```python
from build123d import *

# Parameters (mm, degrees)
SKETCH1_R           = 29
BOSS_EXTRUDE1_DEPTH = 3
SKETCH3_R           = 4
BOSS_EXTRUDE2_DEPTH = 4
SKETCH2_R           = 1.9
CUT_EXTRUDE1_DEPTH  = 42.605288125
SKETCH6_R           = 1.4
CUT_EXTRUDE3_DEPTH  = 10
SKETCH7_R           = 1.4
CUT_EXTRUDE4_DEPTH  = 10
CUT_EXTRUDE5_START  = -10
CUT_EXTRUDE5_DEPTH  = 10
SKETCH4_R           = 1.4
CUT_EXTRUDE7_DEPTH  = 10


with BuildPart() as part:
    # Sketch1 → Boss-Extrude1 (new body)
    with BuildSketch(Plane(origin=(0, 0, 0), x_dir=(1, 0, 0), z_dir=(0, 1, 0))):
        with Locations(Location((0, 0, 0), (0, 0, 270))):
            Circle(SKETCH1_R)
    extrude(amount=BOSS_EXTRUDE1_DEPTH)

    # Sketch3 → Boss-Extrude2 (add)
    with BuildSketch(Plane.XZ):
        with Locations(Location((0, 0, 0), (0, 0, 90))):
            Circle(SKETCH3_R)
    extrude(amount=BOSS_EXTRUDE2_DEPTH)

    # Sketch2 → Cut-Extrude1 (cut, through all)
    with BuildSketch(Plane(origin=(0, 3, 0), x_dir=(1, 0, 0), z_dir=(0, 1, 0))):
        with Locations(Location((0, 0, 0), (0, 0, 270))):
            Circle(SKETCH2_R)
    extrude(amount=-CUT_EXTRUDE1_DEPTH, mode=Mode.SUBTRACT)

    # Sketch6 → Cut-Extrude3 (cut)
    with BuildSketch(Plane(origin=(0, 3, 0), x_dir=(1, 0, 0), z_dir=(0, 1, 0))):
        with Locations(Location((26, 0, 0), (0, 0, 270))):
            Circle(SKETCH6_R)
        with Locations(Location((-26, 0, 0), (0, 0, 270))):
            Circle(SKETCH6_R)
    extrude(amount=-CUT_EXTRUDE3_DEPTH, mode=Mode.SUBTRACT)

    # Sketch7 → Cut-Extrude4 (cut)
    with BuildSketch(Plane(origin=(0, 3, 0), x_dir=(1, 0, 0), z_dir=(0, 1, 0))):
        with Locations(Location((-10, 21.451657064, 0), (0, 0, 270))):
            Circle(SKETCH7_R)
        with Locations(Location((10, 21.451657064, 0), (0, 0, 270))):
            Circle(SKETCH7_R)
    extrude(amount=-CUT_EXTRUDE4_DEPTH, mode=Mode.SUBTRACT)

    # Sketch7_3 → Cut-Extrude5 (cut)
    with BuildSketch(Plane(origin=(0, 3, 0), x_dir=(1, 0, 0), z_dir=(0, 1, 0)).offset(CUT_EXTRUDE5_START)):
        with BuildLine():
            Line((-14, 25.396850198), (0, 25.396850198))
            Line((0, 25.396850198), (0, 29))
            ThreePointArc((0, 29), (-7.228116776, 28.08477039), (-14, 25.396850198))
        make_face()
        with BuildLine():
            Line((0, 29), (0, 25.396850198))
            Line((0, 25.396850198), (14, 25.396850198))
            ThreePointArc((14, 25.396850198), (7.228116776, 28.08477039), (0, 29))
        make_face()
    extrude(amount=CUT_EXTRUDE5_DEPTH, mode=Mode.SUBTRACT)

    # Sketch4 → Cut-Extrude7 (cut)
    with BuildSketch(Plane(origin=(0, 3, 0), x_dir=(1, 0, 0), z_dir=(0, 1, 0))):
        with Locations(Location((-5, -22.025954195, 0), (0, 0, 270))):
            Circle(SKETCH4_R)
        with Locations(Location((5, -22.025954195, 0), (0, 0, 270))):
            Circle(SKETCH4_R)
    extrude(amount=-CUT_EXTRUDE7_DEPTH, mode=Mode.SUBTRACT)


solid = part.part
```
Source: CAD feature listing. Evaluate the final solid. Frame: model axes, mm. A direction names the side the tool comes from. Give positions to 0.01 mm unless a question says otherwise; leave off trailing zeros. Order: outer loops, then holes, each group sorted by start corner. A loop starts at its lowest first (then second) coordinate and runs counter-clockwise, first axis right, second up.
(1) Section query D-D (y = -3). Return the cut outline in (x, z).
(2) Section query A-A (z = 0). Return the cut outline in (x, y), plus the area to 3 significant figures.
(3) Contact query for flat-ended pins moving along their axis: P1, Ø3.5, axis at x = 5, z = 22.03, coming from the -Y side; P2, Ø3.5, axis at x = -26, z = 0, coming from the +Y side; P3, Ø2, axis at y = 0, z = -6, coming from the +X side; P4, Ø3, axis at x = 5, y = -2, coming from the +Z side. Output: stop coordinate, or through.
(4) Section query C-C (x = 5). Return the cut outline in (y, z).
(5) Access query for faces 1 (the face through (5.062, 1.521, 20.627)), 2 (the face through (3.905, -1.972, -0.867)). Directions: +Z, -Z, +X, -X, +Y, -Y. A direction counts if a zero-diameter tool reaches every point of the face in a straight line with its end or side. Return the directions, or none.
(6) Pull-direction query (X, two-part tool) for faces 3 (the face through (0, 0, -5)), 4 (the face through (-0.728, -0.451, 1.755)), 5 (the face through (-1.07, 1.48, 28.98)); classes: +X half, -X half, draft (parallel to the pull), parting line (faces both ways), or undercut.
(7) Section query B-B (y = 1.5). Return the cut outline in (x, z), plus the area to 3 significant figures.
(8) Material intervals for line 1 along X through (y, z) = (2.1, 0); line 2 along X through (y, z) = (-2.5, 0); line 3 along Y through (x, z) = (13.5, 22), sorted ascending.
Outcome:
1. outline: circle Ø8 at (0, 0); hole circle Ø3.8 at (0, 0)
2. outline: (-29, 0) - (-27.4, 0) - (-27.4, 3) - (-29, 3) - close; (-24.6, 0) - (-4, 0) - (-4, -4) - (-1.9, -4) - (-1.9, 3) - (-24.6, 3) - close; (1.9, -4) - (4, -4) - (4, 0) - (24.6, 0) - (24.6, 3) - (1.9, 3) - close; (27.4, 0) - (29, 0) - (29, 3) - (27.4, 3) - close
2. area: 163 mm2
3. P1: stops at y = 0
3. P2: stops at y = 3
3. P3: stops at x = 28.57
3. P4: stops at z = 1.94
4. outline: (0, -25.4) - (3, -25.4) - (3, 20.63) - (0, 20.63) - close; (0, 23.43) - (3, 23.43) - (3, 28.57) - (0, 28.57) - close
5. face 1: +Y, -Y
5. face 2: -Y
6. face 3: draft
6. face 4: undercut
6. face 5: parting line
7. outline: (-14, -25.4) - (14, -25.4) arc R29 ccw (long way) to start; hole circle Ø2.8 at (-26, 0); hole circle Ø2.8 at (-10, -21.45); hole circle Ø2.8 at (-5, 22.03); hole circle Ø3.8 at (0, 0); hole circle Ø2.8 at (5, 22.03); hole circle Ø2.8 at (10, -21.45); hole circle Ø2.8 at (26, 0)
7. area: 2,530 mm2
8. line 1: x = -29 to -27.4, -24.6 to -1.9, 1.9 to 24.6, 27.4 to 29
8. line 2: x = -4 to -1.9, 1.9 to 4
8. line 3: y = 0 to 3
